from build123d import *

# Parameters (mm, degrees)
ESQUISSE1_R             = 12.5
BOSS_EXTRU_1_DEPTH      = 3.5
ESQUISSE2_R             = 10
BOSS_EXTRU_2_DEPTH      = 10.5
ESQUISSE3_R             = 2.5
ENL_V_MAT_EXTRU_1_DEPTH = 7
ESQUISSE4_R             = 7
ENL_V_MAT_EXTRU_2_DEPTH = 2
ESQUISSE5_R             = 8.5
ENL_V_MAT_EXTRU_3_DEPTH = 0.5
ESQUISSE6_R             = 8
ENL_V_MAT_EXTRU_4_DEPTH = 5
CHANFREIN1_SIZE         = 1
CHANFREIN2_SIZE         = 1


with BuildPart() as part:
    # Esquisse1 → Boss.-Extru.1 (new body)
    with BuildSketch(Plane(origin=(0, 0, 0), x_dir=(1, 0, 0), z_dir=(0, 1, 0))):
        with Locations(Location((0, 0, 0), (0, 0, 270))):
            Circle(ESQUISSE1_R)
    extrude(amount=BOSS_EXTRU_1_DEPTH)

    # Esquisse2 → Boss.-Extru.2 (add)
    with BuildSketch(Plane(origin=(0, 3.5, 0), x_dir=(1, 0, 0), z_dir=(0, 1, 0))):
        with Locations(Location((0, 0, 0), (0, 0, 90))):
            Circle(ESQUISSE2_R)
    extrude(amount=BOSS_EXTRU_2_DEPTH)

    # Esquisse3 → Enlèv. mat.-Extru.1 (cut)
    with BuildSketch(Plane.XZ):
        with Locations(Location((0, 0, 0), (0, 0, 270))):
            Circle(ESQUISSE3_R)
    extrude(amount=-ENL_V_MAT_EXTRU_1_DEPTH, mode=Mode.SUBTRACT)

    # Esquisse4 → Enlèv. mat.-Extru.2 (cut)
    with BuildSketch(Plane.XZ.offset(-7)):
        with Locations(Location((0, 0, 0), (0, 0, 270))):
            Circle(ESQUISSE4_R)
    extrude(amount=-ENL_V_MAT_EXTRU_2_DEPTH, mode=Mode.SUBTRACT)

    # Esquisse5 → Enlèv. mat.-Extru.3 (cut)
    with BuildSketch(Plane.XZ.offset(-9)):
        with Locations(Location((0, 0, 0), (0, 0, 270))):
            Circle(ESQUISSE5_R)
    extrude(amount=-ENL_V_MAT_EXTRU_3_DEPTH, mode=Mode.SUBTRACT)

    # Esquisse6 → Enlèv. mat.-Extru.4 (cut)
    with BuildSketch(Plane(origin=(0, 14, 0), x_dir=(1, 0, 0), z_dir=(0, 1, 0))):
        with Locations(Location((0, 0, 0), (0, 0, 270))):
            Circle(ESQUISSE6_R)
    extrude(amount=-ENL_V_MAT_EXTRU_4_DEPTH, mode=Mode.SUBTRACT)

    # Chanfrein1
    chanfrein1_edges = [part.edges().sort_by_distance(p)[0] for p in [
        (0, 3.5, -12.5),
    ]]
    chamfer(chanfrein1_edges, length=CHANFREIN1_SIZE)

    # Chanfrein2
    chanfrein2_edges = [part.edges().sort_by_distance(p)[0] for p in [
        (0, 0, -12.5),
    ]]
    chamfer(chanfrein2_edges, length=CHANFREIN2_SIZE)


solid = part.part
Work out the finished part from the listing and answer in its coordinate system (mm). A direction names the side the tool comes from. Give positions to 0.01 mm unless a question says otherwise; leave off trailing zeros. Loops run counter-clockwise (first coordinate to the right, second up) from the corner with the lowest first, then second, coordinate; pieces in that order, holes last. Notation, with made-up numbers: (20.5, 66.5) -> (66.5, 66.5) arc R24 cw to (66.5, 90.5) -> close; hole circle Ø8 at (64, 38). An arc over 180 degrees is marked (long way). Use a Markdown table: item, result. Add a question column.
1) The part is cut by section C-C, the plane y = 4.5. Determine the outline of the cut face in (x, z).
2) The part is cut by section D-D, the plane y = 10.5. Determine the outline of the cut face in (x, z).
3) The part is cut by section B-B, the plane z = 0. Determine the outline of the cut face in (x, y), plus the area to 3 significant figures.
4) Consider line 1 along X through (y, z) = (8.05, 0); line 2 along X through (y, z) = (9.3, 0); line 3 along Y through (x, z) = (-6, 0). Determine where each line is inside the solid, lowest interval first.
5) The part is cut by section A-A, the plane x = 0. Determine the outline of the cut face in (y, z), plus the area to 3 significant figures.
6) Which of the six approach directions +Z, -Z, +X, -X, +Y, -Y give full straight-line access (tool end or side, diameter ignored) to faces 1 (the cylindrical face through (8.428, 9.246, 1.107)), 2 (the cylindrical face through (-2.44, 3.45, 0.54)), 3 (the cylindrical face through (9.76, 8.68, 2.17))?
7) For a pull along X with two mould halves and no side action, classify faces 4 (the cylindrical face through (-6.834, 7.986, 1.517)), 5 (the flat face through (3, 0, 0)), 6 (the cylindrical face through (3.755, 1.74, 11.923)), 7 (the flat face through (0, 7, -3)) as +X half, -X half, draft (parallel to the pull), parting line (faces both ways), or undercut.
8) Each of these flat-tipped pins is pushed along its axis until it touches: P1, Ø2, axis at x = -8.5, y = 12.5, coming from the +Z side; P2, Ø2, axis at y = 11, z = 0, coming from the -X side; P3, Ø5, axis at x = -9.5, y = 11, coming from the -Z side. Where does it stop, or does it pass through?
Reported:
| question | item | result |
|---|---|---|
| 1 | outline | circle Ø20 at (0, 0); hole circle Ø5 at (0, 0) |
| 2 | outline | circle Ø20 at (0, 0); hole circle Ø16 at (0, 0) |
| 3 | outline | (-12.5, 1) -> (-11.5, 0) -> (-2.5, 0) -> (-2.5, 7) -> (-7, 7) -> (-7, 9) -> (-8.5, 9) -> (-8.5, 9.5) -> (-8, 9.5) -> (-8, 14) -> (-10, 14) -> (-10, 3.5) -> (-11.5, 3.5) -> (-12.5, 2.5) -> close; (2.5, 0) -> (11.5, 0) -> (12.5, 1) -> (12.5, 2.5) -> (11.5, 3.5) -> (10, 3.5) -> (10, 14) -> (8, 14) -> (8, 9.5) -> (8.5, 9.5) -> (8.5, 9) -> (7, 9) -> (7, 7) -> (2.5, 7) -> close |
| 3 | area | 152 mm^2 |
| 4 | line 1 | x = -10 to -7, 7 to 10 |
| 4 | line 2 | x = -10 to -8.5, 8.5 to 10 |
| 4 | line 3 | y = 0 to 7 |
| 5 | outline | (0, -11.5) -> (1, -12.5) -> (2.5, -12.5) -> (3.5, -11.5) -> (3.5, -10) -> (14, -10) -> (14, -8) -> (9.5, -8) -> (9.5, -8.5) -> (9, -8.5) -> (9, -7) -> (7, -7) -> (7, -2.5) -> (0, -2.5) -> close; (0, 2.5) -> (7, 2.5) -> (7, 7) -> (9, 7) -> (9, 8.5) -> (9.5, 8.5) -> (9.5, 8) -> (14, 8) -> (14, 10) -> (3.5, 10) -> (3.5, 11.5) -> (2.5, 12.5) -> (1, 12.5) -> (0, 11.5) -> close |
| 5 | area | 152 mm^2 |
| 6 | face 1 | none |
| 6 | face 2 | +Y, -Y |
| 6 | face 3 | +Y |
| 7 | face 4 | undercut |
| 7 | face 5 | draft |
| 7 | face 6 | parting line |
| 7 | face 7 | undercut |
| 8 | P1 | stops at z = 6.61 |
| 8 | P2 | stops at x = -10 |
| 8 | P3 | stops at z = -7.14 |
